For this review, use the dimensioned drawing (mm, ordinates from the lowest corner) and the shaded views. Coordinates: 2 decimals unless noted, no trailing zeros. Write each loop counter-clockwise with the first axis right and the second up, starting at its lowest first coordinate (ties: lowest second). Pieces come first, ordered by that corner, then holes. Notation, with made-up numbers: M -4,15.25 L 9,15.25 A22 ccw 9,52.25 Z; hole C -27,58 d6. An arc over 180 degrees is marked long. Return JSON: item names as keys, results as strings. Group by question number.
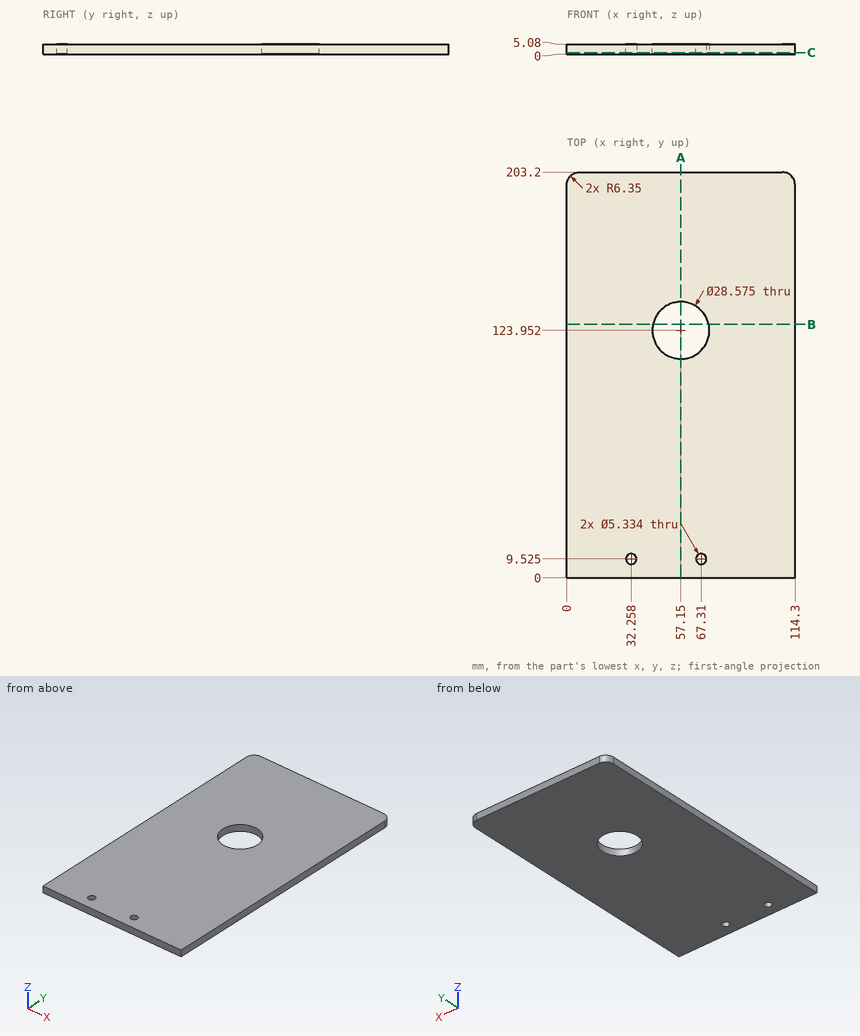
Item 1: Add section C-C (z = 0.8). Count the separate pieces of the cut face and the enclosed holes in it, plus the area to 3 significant figures.
Item 2: Add section A-A (x = 57.15). Write out the cut boundary in (y, z).
Item 3: For line 1 (Y direction, x = 57.15, z = 3); line 2 (Y direction, x = 67.31, z = 2.75); line 3 (Y direction, x = 45, z = 4.9), list the stretches that pass through material, from the lowest coordinate up.
Item 4: Add section B-B (y = 127). Write out the cut boundary in (x, z).
Item 5: For pin 1 (23 mm diameter, centred on x = 57.15, y = 123.952, fed in from -Z), flat-tipped, find the tip position at first contact; note if it passes through.
Geometry check:
{
 "1": {"separate pieces": "1", "enclosed holes": "3", "area": "22,500 mm^2"},
 "2": {"outline": "M 0,0 L 109.66,0 L 109.66,5.08 L 0,5.08 Z; M 138.24,0 L 203.2,0 L 203.2,5.08 L 138.24,5.08 Z"},
 "3": {"line 1": "0 to 109.66, 138.24 to 203.2", "line 2": "0 to 6.86, 12.19 to 113.91, 134 to 203.2", "line 3": "0 to 116.43, 131.47 to 203.2"},
 "4": {"outline": "M 0,0 L 43.19,0 L 43.19,5.08 L 0,5.08 Z; M 71.11,0 L 114.3,0 L 114.3,5.08 L 71.11,5.08 Z"},
 "5": {"pin 1": "through"}
}
